Work out the finished part from the listing and answer in its coordinate system (mm). Round coordinates to 2 decimals unless told otherwise and drop trailing zeros. Loops run counter-clockwise (first coordinate to the right, second up) from the corner with the lowest first, then second, coordinate; pieces in that order, holes last.
```python
from build123d import *

# Parameters (mm, degrees)
SKETCH1_W           = 253
SKETCH1_H           = 50
BOSS_EXTRUDE1_DEPTH = 17.5
SKETCH2_W           = 22
SKETCH2_H           = 45
CUT_EXTRUDE1_DEPTH  = 10
SKETCH3_W           = 14.5
SKETCH3_H           = 20
CUT_EXTRUDE2_DEPTH  = 17.5
LPATTERN1_COUNT     = 10
LPATTERN1_PITCH     = 25


with BuildPart() as part:
    # Sketch1 → Boss-Extrude1 (new body)
    with BuildSketch(Plane(origin=(0, 0, 0), x_dir=(1, 0, 0), z_dir=(0, 1, 0))):
        with Locations((126.5, -25)):
            Rectangle(SKETCH1_W, SKETCH1_H)
    extrude(amount=BOSS_EXTRUDE1_DEPTH)

    # Sketch2 → Cut-Extrude1 (cut)
    with BuildSketch(Plane(origin=(0, 17.5, 0), x_dir=(1, 0, 0), z_dir=(0, 1, 0))):
        with Locations((14, -25)):
            Rectangle(SKETCH2_W, SKETCH2_H)
    cut_extrude1 = extrude(amount=-CUT_EXTRUDE1_DEPTH, mode=Mode.SUBTRACT)

    # Sketch3 → Cut-Extrude2 (cut)
    with BuildSketch(Plane(origin=(0, 17.5, 0), x_dir=(1, 0, 0), z_dir=(0, 1, 0))):
        with Locations((17.75, -25)):
            Rectangle(SKETCH3_W, SKETCH3_H)
    cut_extrude2 = extrude(amount=-CUT_EXTRUDE2_DEPTH, mode=Mode.SUBTRACT)

    # LPattern1: Cut-Extrude1, Cut-Extrude2 ×10
    with Locations(*[(i * LPATTERN1_PITCH, 0, 0) for i in range(1, LPATTERN1_COUNT)]):
        add(cut_extrude1, mode=Mode.SUBTRACT)
        add(cut_extrude2, mode=Mode.SUBTRACT)


solid = part.part
```
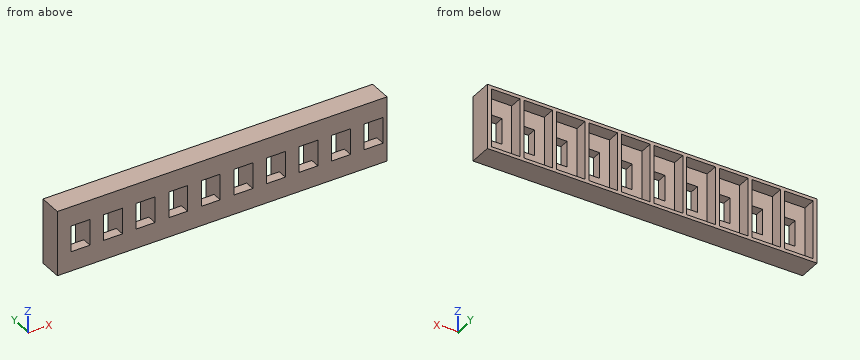
1. Consider probe 1 along Z at (x, y) = (196, 2.25); probe 2 along Z at (x, y) = (139, 16.75); probe 3 along Y at (x, z) = (156.5, 29.5). Determine where each line is inside the solid, lowest interval first.
Answer key:
probe 1: z = 0 to 15, 35 to 50
probe 2: z = 0 to 2.5, 47.5 to 50
probe 3: y = 0 to 7.5
2. Find section B-B (z = 22.5). Give the number of separate pieces and of enclosed holes in the cut face, then the cut area to 3 significant figures.
Answer key:
separate pieces: 11
enclosed holes: 0
area: 1,140 mm2
3. Find section A-A (x = 19). Write down the section's boundary in (y, z), then the cut area to 3 significant figures.
Answer key:
outline: (0, 0) - (17.5, 0) - (17.5, 2.5) - (7.5, 2.5) - (7.5, 15) - (0, 15) - close; (0, 35) - (7.5, 35) - (7.5, 47.5) - (17.5, 47.5) - (17.5, 50) - (0, 50) - close
area: 275 mm2
4. Given pin 1 (17.5 mm diameter, centred on x = 238.5, z = 29.5, fed in from +Y), flat-ended and moving along its own axis, determine where the tip first touches the part or whether it passes through.
Answer key:
pin 1: stops at y = 7.5
